```python
from build123d import *

# Parameters (mm, degrees)
SKETCH1_W           = 230.8225
SKETCH1_H           = 12.7
BOSS_EXTRUDE1_DEPTH = 12.7
SKETCH2_W           = 6.35
SKETCH2_H           = 6.35
CUT_EXTRUDE1_DEPTH  = 6.35
FILLET1_R           = 1.5875


with BuildPart() as part:
    # Sketch1 → Boss-Extrude1 (new body)
    with BuildSketch(Plane(origin=(0, 0, 0), x_dir=(1, 0, 0), z_dir=(0, 1, 0))):
        with Locations((115.41125, 6.35)):
            Rectangle(SKETCH1_W, SKETCH1_H)
    extrude(amount=BOSS_EXTRUDE1_DEPTH)

    # Sketch2 → Cut-Extrude1 (cut)
    with BuildSketch(Plane(origin=(0, 12.7, 0), x_dir=(1, 0, 0), z_dir=(0, 1, 0))):
        with Locations((221.2975, 6.35)):
            Rectangle(SKETCH2_W, SKETCH2_H)
        with Locations((9.525, 6.35)):
            Rectangle(SKETCH2_W, SKETCH2_H)
    extrude(amount=-CUT_EXTRUDE1_DEPTH, mode=Mode.SUBTRACT)

    # Fillet1
    fillet1_edges = [part.edges().sort_by_distance(p)[0] for p in [
        (230.8225, 12.7, -6.35),
        (115.41125, 12.7, 0),
        (218.1225, 12.7, -6.35),
        (221.2975, 12.7, -3.175),
        (224.4725, 12.7, -6.35),
        (221.2975, 12.7, -9.525),
        (12.7, 12.7, -6.35),
        (9.525, 12.7, -9.525),
        (6.35, 12.7, -6.35),
        (9.525, 12.7, -3.175),
        (0, 12.7, -6.35),
        (115.41125, 0, 0),
        (230.8225, 0, -6.35),
        (115.41125, 0, -12.7),
        (0, 0, -6.35),
        (0, 6.35, 0),
        (230.8225, 6.35, 0),
        (230.8225, 6.35, -12.7),
        (0, 6.35, -12.7),
        (115.41125, 12.7, -12.7),
    ]]
    fillet(fillet1_edges, radius=FILLET1_R - 0.0001)  # a hair under: the kernel refuses the full size


solid = part.part
```
Can you work these out from the model? Positions are in its coordinate system, mm. A direction names the side the tool comes from. Give positions to 0.01 mm unless a question says otherwise; leave off trailing zeros. Loops run counter-clockwise (first coordinate to the right, second up) from the corner with the lowest first, then second, coordinate; pieces in that order, holes last. Notation, with made-up numbers: M 60,80.25 L 74,80.25 A28 cw 74,106.25 Z; hole C -16,75 d6. An arc over 180 degrees is marked long. One line per question, with ' | ' between items. Start each with the question number.
Q1. If we section it at B-B (z = -7.25): Please give me the cut outline in (x, y), plus the area to 3 significant figures.
Q2. For faces 4 (the flat face through (12.7, 9, -6)), 5 (the flat face through (114, 0, -6)), which set-ups out of +Z, -Z, +X, -X, +Y, -Y let a thin tool reach every point of the face, with its end or its side?
Q3. For pin 1 Ø7 at (x, z) = (221.5, -6) entering from +Y; pin 2 Ø1.9 at (x, z) = (10, -5) entering from +Y, each with a flat end and sliding along its axis, tell me the tip position at first contact or that it passes through.
Q4. If we section it at A-A (y = 9): State how many separate pieces and enclosed holes the cut face has, plus the area to 3 significant figures.
Q5. If we mould it in two halves opening along Z, with no side actions, what happens to faces 1 (the flat face through (230.822, 6, -6)), 2 (the flat face through (114, 6, 0)), 3 (the flat face through (221, 6.35, -6))? For each: +Z half, -Z half, draft (parallel to the pull), parting line (faces both ways), or undercut.
Q6. If I drill on line 1 (X direction, y = 9.5, z = -4); line 2 (Y direction, x = 105, z = -1.5), over which ranges is the centre line in solid material (lowest first)? Write a range as from..to.
Computed:
1) outline: M 0,1.59 A1.59 ccw 1.59,0 L 229.24,0 A1.59 ccw 230.82,1.59 L 230.82,11.11 A1.59 ccw 229.24,12.7 L 226.06,12.7 A1.59 ccw 224.47,11.11 L 224.47,6.35 L 218.12,6.35 L 218.12,11.11 A1.59 ccw 216.54,12.7 L 14.29,12.7 A1.59 ccw 12.7,11.11 L 12.7,6.35 L 6.35,6.35 L 6.35,11.11 A1.59 ccw 4.76,12.7 L 1.59,12.7 A1.59 ccw 0,11.11 Z | area: 2,850 mm²
2) face 4: +Y | face 5: +Z, -Z, +X, -X, -Y
3) pin 1: stops at y = 12.41 | pin 2: stops at y = 6.35
4) separate pieces: 1 | enclosed holes: 2 | area: 2,850 mm²
5) face 1: draft | face 2: +Z half | face 3: undercut
6) line 1: x = 0..6.35, 12.7..218.12, 224.47..230.82 | line 2: y = 0..12.7
